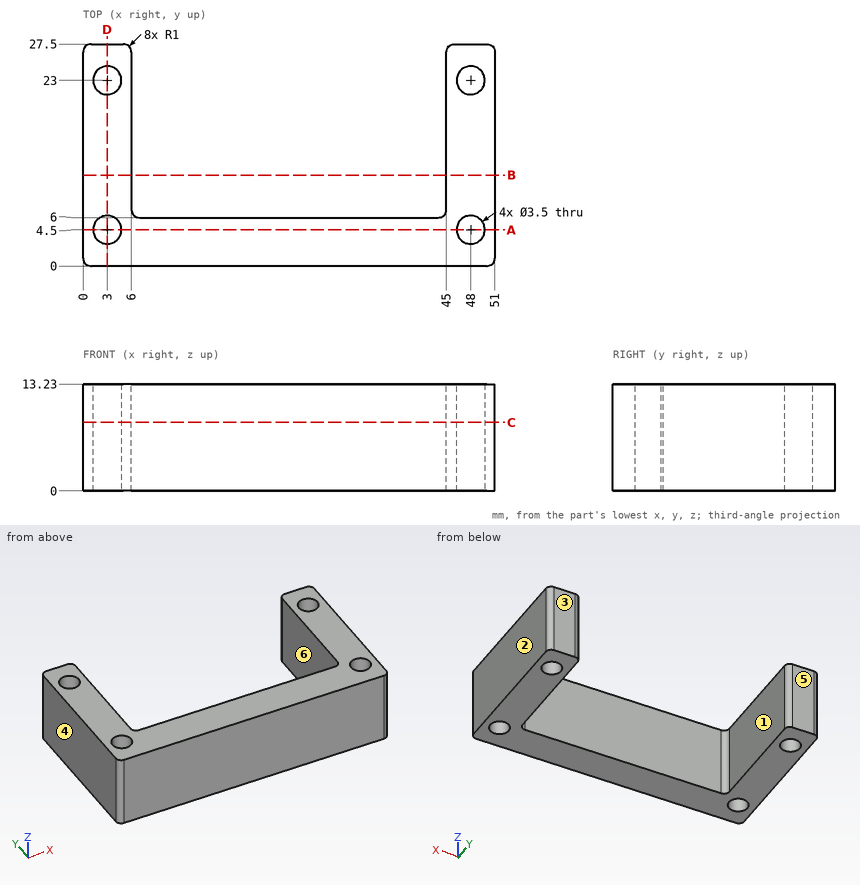
Could you check a few things on this drawing? It's one solid part, dimensions in mm from its lowest x, y, z. A direction names the side the tool comes from. Coordinates: 2 decimals unless noted, no trailing zeros. Order: outer loops, then holes, each group sorted by start corner. A loop starts at its lowest first (then second) coordinate and runs counter-clockwise, first axis right, second up. Notation, with made-up numbers: M 0,81 L 38,81 A26 cw 38,118 Z; hole C 59,3.5 d9. An arc over 180 degrees is marked long. Use a Markdown table: item, result. Add a question column.
Q1. I want a section at B-B on y = 11.25. List the corners of the cut face in (x, z) for me, then the cut area to 3 significant figures.
Q2. I'm going to push flat-ended pins straight in: pin 1 (5.5 mm diameter, centred on x = 3, y = 4.5, fed in from -Z); pin 2 (4 mm diameter, centred on x = 30.5, z = 9.5, fed in from +Y). Where does each tip first touch, or does it pass through?
Q3. I want a section at D-D on x = 3. List the corners of the cut face in (y, z) for me.
Q4. I want a section at A-A on y = 4.5. List the corners of the cut face in (x, z) for me.
Q5. If I drill on L1, parallel to Y at x = 3, z = 8; L2, parallel to X at y = 7.5, z = 9.75; L3, parallel to Y at x = 4.5, z = 2, over which ranges is the centre line in solid material (lowest first)?
Q6. Which directions (+Z, -Z, +X, -X, +Y, -Y) give clear straight access to the entire face, cutting with the end or side of a thin tool? Please do the marked faces 5 and 6.
Q7. We'd pull the mould along X, two halves only. Please class the marked faces 1, 2, 3 and 4: pulls with the +X half, pulls with the -X half, needs draft (parallel to the pull), parting line crosses it, or undercut.
Q8. I want a section at C-C on z = 8.5. List the corners of the cut face in (x, y) for me, then the cut area to 3 significant figures.
Checked values:
| question | item | result |
|---|---|---|
| 1 | outline | M 0,0 L 6,0 L 6,13.23 L 0,13.23 Z; M 45,0 L 51,0 L 51,13.23 L 45,13.23 Z |
| 1 | area | 159 mm² |
| 2 | pin 1 | z = 0 |
| 2 | pin 2 | y = 6 |
| 3 | outline | M 0,0 L 2.75,0 L 2.75,13.23 L 0,13.23 Z; M 6.25,0 L 21.25,0 L 21.25,13.23 L 6.25,13.23 Z; M 24.75,0 L 27.5,0 L 27.5,13.23 L 24.75,13.23 Z |
| 4 | outline | M 0,0 L 1.25,0 L 1.25,13.23 L 0,13.23 Z; M 4.75,0 L 46.25,0 L 46.25,13.23 L 4.75,13.23 Z; M 49.75,0 L 51,0 L 51,13.23 L 49.75,13.23 Z |
| 5 | L1 | 0 to 2.75, 6.25 to 21.25, 24.75 to 27.5 |
| 5 | L2 | 0 to 6, 45 to 51 |
| 5 | L3 | 0 to 3.6, 5.4 to 22.1, 23.9 to 27.5 |
| 6 | face 5 | +Z, -Z, +X, -X, +Y |
| 6 | face 6 | +Z, -Z, +Y |
| 7 | face 1 | undercut |
| 7 | face 2 | pulls with the +X half |
| 7 | face 3 | needs draft |
| 7 | face 4 | pulls with the -X half |
| 8 | outline | M 0,1 A1 ccw 1,0 L 50,0 A1 ccw 51,1 L 51,26.5 A1 ccw 50,27.5 L 46,27.5 A1 ccw 45,26.5 L 45,7 A1 cw 44,6 L 7,6 A1 cw 6,7 L 6,26.5 A1 ccw 5,27.5 L 1,27.5 A1 ccw 0,26.5 Z; hole C 3,4.5 d3.5; hole C 3,23 d3.5; hole C 48,4.5 d3.5; hole C 48,23 d3.5 |
| 8 | area | 525 mm² |
